from build123d import *

# Parameters (mm, degrees)
BOSS_EXTRUDE2_DEPTH = 6.35
SKETCH3_R           = 4.25
CUT_EXTRUDE1_DEPTH  = 53.294538816
FILLET1_R           = 1


with BuildPart() as part:
    # Sketch2 → Boss-Extrude2 (new body)
    with BuildSketch(Plane(origin=(0, 0, 0), x_dir=(1, 0, 0), z_dir=(0, 1, 0))):
        Polygon((46.7, -22.660677173), (46.7, 15.560677173), (24.2, 15.560677173), (24.2, 22.660677173), (-24.2, 22.660677173), (-24.2, 15.560677173), (-46.7, 15.560677173), (-46.7, -22.660677173), align=None)
    extrude(amount=BOSS_EXTRUDE2_DEPTH)

    # Sketch3 → Cut-Extrude1 (cut, through all)
    with BuildSketch(Plane(origin=(0, 6.35, 0), x_dir=(1, 0, 0), z_dir=(0, 1, 0))):
        with Locations(Location((-21.05, -4.225241458, 0), (0, 0, 270))):
            Circle(SKETCH3_R)
        with Locations(Location((21.05, -4.275241458, 0), (0, 0, 270))):
            Circle(SKETCH3_R)
    extrude(amount=-CUT_EXTRUDE1_DEPTH, mode=Mode.SUBTRACT)

    # Fillet1
    fillet1_edges = [part.edges().sort_by_distance(p)[0] for p in [
        (-46.7, 3.175, 22.660677173),
        (-46.7, 3.175, -15.560677173),
        (-24.2, 3.175, -15.560677173),
        (-24.2, 3.175, -22.660677173),
        (24.2, 3.175, -22.660677173),
        (24.2, 3.175, -15.560677173),
        (46.7, 3.175, -15.560677173),
        (46.7, 3.175, 22.660677173),
    ]]
    fillet(fillet1_edges, radius=FILLET1_R)


solid = part.part
Can you work these out from the model? Positions are in its coordinate system, mm. A direction names the side the tool comes from. Round coordinates to 2 decimals unless told otherwise and drop trailing zeros. Order: outer loops, then holes, each group sorted by start corner. A loop starts at its lowest first (then second) coordinate and runs counter-clockwise, first axis right, second up. Notation, with made-up numbers: (64.25, -33) - (80.25, -33) arc R14 cw to (80.25, -16) - close; hole circle Ø9 at (72.25, 49.5). An arc over 180 degrees is marked (long way). Answer in a Markdown table with one row per item.
(1) Suppose I cut it at B-B, the plane y = 1.25. Please give me the cut outline in (x, z), plus the area to 3 significant figures.
From the geometry:
| item | result |
|---|---|
| outline | (-46.7, -14.56) arc R1 ccw to (-45.7, -15.56) - (-25.2, -15.56) arc R1 cw to (-24.2, -16.56) - (-24.2, -21.66) arc R1 ccw to (-23.2, -22.66) - (23.2, -22.66) arc R1 ccw to (24.2, -21.66) - (24.2, -16.56) arc R1 cw to (25.2, -15.56) - (45.7, -15.56) arc R1 ccw to (46.7, -14.56) - (46.7, 21.66) arc R1 ccw to (45.7, 22.66) - (-45.7, 22.66) arc R1 ccw to (-46.7, 21.66) - close; hole circle Ø8.5 at (-21.05, 4.23); hole circle Ø8.5 at (21.05, 4.28) |
| area | 3,800 mm2 |
(2) Suppose I cut it at A-A, the plane x = -21.05. Please give me the cut outline in (y, z), plus the area to 3 significant figures.
From the geometry:
| item | result |
|---|---|
| outline | (0, -22.66) - (6.35, -22.66) - (6.35, -0.02) - (0, -0.02) - close; (0, 8.48) - (6.35, 8.48) - (6.35, 22.66) - (0, 22.66) - close |
| area | 234 mm2 |
(3) For P1, Ø7.5, axis at x = -21.05, z = 4.23, coming from the -Y side; P2, Ø3, axis at x = -36.5, y = 4, coming from the -Z side; P3, Ø2.5, axis at y = 2.5, z = -18, coming from the -X side, each with a flat end and sliding along its axis, tell me the tip position at first contact or that it passes through.
From the geometry:
| item | result |
|---|---|
| P1 | passes through |
| P2 | stops at z = -15.56 |
| P3 | stops at x = -24.2 |
(4) Suppose I cut it at D-D, the plane x = 22. Please give me the cut outline in (y, z).
From the geometry:
| item | result |
|---|---|
| outline | (0, -22.66) - (6.35, -22.66) - (6.35, 0.13) - (0, 0.13) - close; (0, 8.42) - (6.35, 8.42) - (6.35, 22.66) - (0, 22.66) - close |
(5) Suppose I cut it at C-C, the plane z = 7.5. Please give me the cut outline in (x, y), plus the area to 3 significant figures.
From the geometry:
| item | result |
|---|---|
| outline | (-46.7, 0) - (-23.76, 0) - (-23.76, 6.35) - (-46.7, 6.35) - close; (-18.34, 0) - (18.28, 0) - (18.28, 6.35) - (-18.34, 6.35) - close; (23.82, 0) - (46.7, 0) - (46.7, 6.35) - (23.82, 6.35) - close |
| area | 524 mm2 |
(6) Please list where these lines run through material, in increasing order: L1, parallel to X at y = 2, z = 3; L2, parallel to Z at x = -32.5, y = 2.5; L3, parallel to Z at x = -22, y = 4.5. Write a range as from..to.
From the geometry:
| item | result |
|---|---|
| L1 | x = -46.7..-25.12, -16.98..17, 25.1..46.7 |
| L2 | z = -15.56..22.66 |
| L3 | z = -22.66..0.08, 8.37..22.66 |
(7) If we mould it in two halves opening along Z, with no side actions, what happens to faces 1 (the face through (25.264, 3.219, 3.722)), 2 (the face through (-35, 3, -15.561)), 3 (the face through (-23, 3, 8)), 4 (the face through (-1, 3, 22.661))? For each: released by +Z, released by -Z, zero draft, split by the parting line, or undercut.
From the geometry:
| item | result |
|---|---|
| face 1 | undercut |
| face 2 | released by -Z |
| face 3 | undercut |
| face 4 | released by +Z |
(8) Which directions (+Z, -Z, +X, -X, +Y, -Y) give clear straight access to the entire face, cutting with the end or side of a thin tool? Please do faces 5 (the face through (-1, 0, 0)), 6 (the face through (24.2, 3, -19)), 7 (the face through (-24.2, 3, -19)).
From the geometry:
| item | result |
|---|---|
| face 5 | +Z, -Z, +X, -X, -Y |
| face 6 | -Z, +X, +Y, -Y |
| face 7 | -Z, -X, +Y, -Y |
